Model file for the job. Use its own axes, mm. A direction names the side the tool comes from. Coordinates: 2 decimals unless noted, no trailing zeros. Order: outer loops, then holes, each group sorted by start corner. A loop starts at its lowest first (then second) coordinate and runs counter-clockwise, first axis right, second up. Notation, with made-up numbers: M -34,15 L -16,15 A29 ccw -16,44 Z; hole C -4.5,63.5 d10. An arc over 180 degrees is marked long. Return JSON: item names as keys, results as strings.
```python
from build123d import *

# Parameters (mm, degrees)
F0_W      = 1795
F0_H      = 1300
F1_DEPTH  = 300
F2_W      = 165
F2_H      = 635
F2_W_2    = 300
F2_H_2    = 135
F2_W_3    = 897.5
F2_H_3    = 50
F2_W_4    = 490
F2_H_4    = 20
F3_DEPTH  = 300
F4_T      = -40
F5_W      = 80
F5_H      = 150
F5_W_2    = 15
F5_H_2    = 40
F5_W_3    = 20
F5_H_3    = 20
F6_DEPTH  = 260
F8_DEPTH  = 25
F10_DEPTH = 50
F12_DEPTH = 260
F14_DEPTH = 400
F16_DEPTH = 1630


with BuildPart() as f1:
    # F0 (on Top) → F1 (new body)
    with BuildSketch(Plane.XY):
        Rectangle(F0_W, F0_H)
    extrude(amount=F1_DEPTH)

    # F2 (on face) → F3 (cut)
    with BuildSketch(Plane(origin=(0, 0, 0), x_dir=(1, 0, 0), z_dir=(0, 0, -1))):
        with Locations((-815, 332.5)):
            Rectangle(F2_W, F2_H)
        with Locations((-747.5, -582.5)):
            Rectangle(F2_W_2, F2_H_2)
        with Locations((448.75, 625)):
            Rectangle(F2_W_3, F2_H_3)
        Polygon((-67.5, -650), (897.5, -650), (897.5, -515), (407.5, -515), (-67.5, -515), align=None)
        with Locations((652.5, -505)):
            Rectangle(F2_W_4, F2_H_4)
    extrude(amount=-F3_DEPTH, mode=Mode.SUBTRACT)

    # F4
    f4_openings = [f1.faces().sort_by_distance(p)[0] for p in [
        (17.505881, -20.736482, 300),
    ]]
    offset(amount=F4_T, openings=f4_openings, kind=Kind.INTERSECTION)

    # F5 (on face) → F6 (join)
    with BuildSketch(Plane.XY.offset(40)):
        Polygon((132.5, 10), (132.5, -560), (147.5, -560), (147.5, 10), (367.5, 10), (367.5, -415), (427.5, -415), (427.5, -560), (437.5, -560), (437.5, -415), (472.5, -415), (472.5, -250), (857.5, -250), (857.5, -235), (382.5, -235), (382.5, 455), (367.5, 455), (367.5, 25), (-92.5, 25), (-92.5, 475), (-107.5, 475), (-107.5, 25), (-557.5, 25), (-557.5, 475), (-572.5, 475), (-572.5, 25), (-692.5, 25), (-692.5, 10), align=None)
        with Locations((422.5, -325)):
            Rectangle(F5_W, F5_H, mode=Mode.SUBTRACT)
        with Locations((-700, 45)):
            Rectangle(F5_W_2, F5_H_2)
        Polygon((-857.5, 215), (-857.5, 205), (-707.5, 205), (-707.5, 165), (-692.5, 165), (-692.5, 205), (-692.5, 215), (-692.5, 275), (-707.5, 275), (-707.5, 215), align=None)
        with Locations((-327.5, -120)):
            Rectangle(F5_W_3, F5_H_3)
    extrude(amount=F6_DEPTH)

    # F7 (on face) → F8 (join)
    with BuildSketch(Plane.XY.offset(300)):
        Polygon((-897.5, -15), (-732.5, -15), (-732.5, -650), (0, -650), (0, -600), (897.5, -600), (897.5, 495), (407.5, 495), (407.5, 515), (-67.5, 515), (-67.5, 650), (-597.5, 650), (-597.5, 515), (-897.5, 515), align=None)
    extrude(amount=F8_DEPTH)

    # F9 (on face) → F10 (join)
    with BuildSketch(Plane.XZ.offset(650)):
        Polygon((-732.5, 480), (-732.5, 325), (0, 325), (0, 480), (-366.25, 846.25), align=None)
    extrude(amount=-F10_DEPTH)

    # F11 (on face) → F12 (join)
    with BuildSketch(Plane.XY.offset(325)):
        Polygon((-897.5, -15), (-732.5, -15), (-732.5, -600), (-692.5, -600), (-542.5, -600), (-542.5, -560), (-692.5, -560), (-692.5, 25), (-857.5, 25), (-857.5, 475), (-557.5, 475), (-557.5, 610), (-107.5, 610), (-107.5, 475), (367.5, 475), (367.5, 455), (857.5, 455), (857.5, -560), (-150, -560), (-150, -600), (0, -600), (897.5, -600), (897.5, 495), (407.5, 495), (407.5, 515), (-67.5, 515), (-67.5, 650), (-597.5, 650), (-597.5, 515), (-897.5, 515), align=None)
    extrude(amount=F12_DEPTH)

    # F13 (on face) → F14 (join)
    with BuildSketch(Plane(origin=(0, -600, 0), x_dir=(-1, 0, 0), z_dir=(0, 1, 0))):
        Polygon((627.5, 585), (366.25, 846.25), (105, 585), align=None)
    extrude(amount=F14_DEPTH)

    # F15 (on face) → F16 (join)
    with BuildSketch(Plane.YZ.offset(897.5)):
        Polygon((-52.5, 1132.5), (-600, 585), (495, 585), align=None)
    extrude(amount=-F16_DEPTH)


solid = f1.part
```
Item 1: 3-axis set-ups, long thin cutter, end or side, ignore diameter. For faces 1 (the flat face through (-816, -15, 288)), 2 (the flat face through (173, 515, 288)), 3 (the flat face through (361, -560, 453)), 4 (the flat face through (-704, -600, 555)): which of +Z, -Z, +X, -X, +Y, -Y reach the whole face in a straight line?
Check result:
{"face 1": "+Z, -Z, -X, -Y", "face 2": "+Z, -Z, +X, +Y", "face 3": "none", "face 4": "+Z, -X, -Y"}
Item 2: Saw through at C-C (y = -454). Write the cut outline in (x, z).
Check result:
{"outline": "M -732.5,0 L 897.5,0 L 897.5,731 L -251,731 L -366.25,846.25 L -481.5,731 L -732.5,731 Z; hole M -692.5,40 L 132.5,40 L 132.5,300 L -692.5,300 Z; hole M -692.5,325 L 857.5,325 L 857.5,585 L -692.5,585 Z; hole M 147.5,40 L 427.5,40 L 427.5,300 L 147.5,300 Z; hole M 437.5,40 L 857.5,40 L 857.5,300 L 437.5,300 Z"}
Item 3: Saw through at A-A (x = -424). Write the cut outline in (y, z).
Check result:
{"outline": "M -650,0 L 650,0 L 650,585 L 610,585 L 610,325 L -600,325 L -600,585 L 495,585 L -52.5,1132.5 L -396.5,788.5 L -650,788.5 Z; hole M -610,40 L 10,40 L 10,300 L -610,300 Z; hole M 25,40 L 610,40 L 610,300 L 25,300 Z"}
Item 4: Pull direction Z, two halves, no side cores. Call faces 5 (the flat face through (422, -324, 300)), 6 (the flat face through (0, -625, 237)): +Z half, -Z half, draft (parallel to the pull), parting line (faces both ways), or undercut.
Check result:
{"face 5": "undercut", "face 6": "draft"}
Item 5: Saw through at D-D (x = 543). Write the cut outline in (y, z), and give its area (3 significant figures).
Check result:
{"outline": "M -600,0 L 495,0 L 495,585 L -52.5,1132.5 L -600,585 Z; hole M -560,40 L -250,40 L -250,300 L -560,300 Z; hole M -560,325 L 455,325 L 455,585 L -560,585 Z; hole M -235,40 L 455,40 L 455,300 L -235,300 Z", "area": "416,000 mm2"}
Item 6: Wall check: line 1 (X direction, y = -51.5, z = 213); line 2 (Y direction, x = 299.5, z = 69); line 3 (Y direction, x = 635, z = 251.5). Give the ranges that are in metal, low to high.
Check result:
{"line 1": "x = -732.5 to -692.5, 132.5 to 147.5, 367.5 to 382.5, 857.5 to 897.5", "line 2": "y = -600 to -560, 10 to 25, 475 to 515", "line 3": "y = -600 to -560, -250 to -235, 455 to 495"}
Item 7: Drop flat-ended pins along their axis: pin 1 Ø10 at (x, z) = (180.5, 552.5) entering from -Y; pin 2 Ø3 at (x, z) = (92.5, 634) entering from -Y; pin 3 Ø10 at (x, y) = (409, -506.5) entering from +Z. Give the stop position or say it passes through.
Check result:
{"pin 1": "stops at y = -600", "pin 2": "stops at y = -552.5", "pin 3": "stops at z = 683.5"}
